from build123d import *

# Parameters (mm, degrees)
SKETCH_1_R          = 2
EXTRUDE_1_DEPTH     = 5
SKETCH_3_W          = 30
SKETCH_3_H          = 2.196813629
EXTRUDE_2_DEPTH     = 10
SKETCH_4_R          = 1.4
CUT_EXTRUDE_2_DEPTH = 20
EXTRUDE_START       = 5.803186371
SKETCH_5_W          = 4
SKETCH_5_H          = 3.6
SKETCH_5_R          = 1.424260765
SKETCH_5_R_2        = 1.4
EXTRUDE_3_DEPTH     = 5.803186371
SKETCH_6_W          = 5.555026764
SKETCH_6_H          = 4.966415056
EXTRUDE_4_DEPTH     = 7
SKETCH_8_R          = 2.9
CUT_EXTRUDE_3_DEPTH = 5
SKETCH_9_R          = 2.2
EXTRUDE_5_DEPTH     = 5
FILLET_1_R          = 1


with BuildPart() as part:
    # 스케치1 → 보스-돌출1 (new, symmetric)
    with BuildSketch(Plane(origin=(0, 0, 0), x_dir=(0, 0, -1), z_dir=(1, 0, 0))):
        Polygon((15, 6.896813629), (-15, 6.896813629), (-15, -1.103186371), (-10.2, -1.103186371), (-10.2, 4.7), (-5, 4.7), (-5, -4), (5, -4), (5, 4.7), (10.2, 4.7), (10.2, -1.103186371), (15, -1.103186371), align=None)
        Circle(SKETCH_1_R, mode=Mode.SUBTRACT)
    extrude(amount=EXTRUDE_1_DEPTH, both=True)

    # 스케치3 → 보스-돌출2 (add, symmetric)
    with BuildSketch(Plane(origin=(0, 0, 0), x_dir=(0, 0, -1), z_dir=(1, 0, 0))):
        with Locations((0, 5.798406814)):
            Rectangle(SKETCH_3_W, SKETCH_3_H)
    extrude(amount=EXTRUDE_2_DEPTH, both=True)

    # 스케치4 → 컷-돌출2 (cut)
    with BuildSketch(Plane(origin=(0, 0, 0), x_dir=(1, 0, 0), z_dir=(0, 1, 0))):
        with Locations(Location((-7, -12, 0), (0, 0, 90))):
            Circle(SKETCH_4_R)
        with Locations(Location((7, -12, 0), (0, 0, 90))):
            Circle(SKETCH_4_R)
        with Locations(Location((7, 12, 0), (0, 0, 90))):
            Circle(SKETCH_4_R)
        with Locations(Location((-7, 12, 0), (0, 0, 90))):
            Circle(SKETCH_4_R)
    extrude(amount=CUT_EXTRUDE_2_DEPTH, mode=Mode.SUBTRACT)

    # 스케치5 → 보스-돌출3 (add)
    # profile 1 of 4: a face of its own
    with BuildSketch(Plane.XZ.offset(-4.7).offset(EXTRUDE_START)):
        with Locations((-7, -12)):
            Rectangle(SKETCH_5_W, SKETCH_5_H)
        with Locations(Location((-7, -12, 0), (0, 0, 90))):
            Circle(SKETCH_5_R, mode=Mode.SUBTRACT)
    # profile 2 of 4: a face of its own
    with BuildSketch(Plane.XZ.offset(-4.7).offset(EXTRUDE_START)):
        with Locations((7, -12)):
            Rectangle(SKETCH_5_W, SKETCH_5_H)
        with Locations(Location((7, -12, 0), (0, 0, 270))):
            Circle(SKETCH_5_R_2, mode=Mode.SUBTRACT)
    # profile 3 of 4: a face of its own
    with BuildSketch(Plane.XZ.offset(-4.7).offset(EXTRUDE_START)):
        with Locations((7, 12)):
            Rectangle(SKETCH_5_W, SKETCH_5_H)
        with Locations(Location((7, 12, 0), (0, 0, 270))):
            Circle(SKETCH_5_R_2, mode=Mode.SUBTRACT)
    # profile 4 of 4: a face of its own
    with BuildSketch(Plane.XZ.offset(-4.7).offset(EXTRUDE_START)):
        with Locations((-7, 12)):
            Rectangle(SKETCH_5_W, SKETCH_5_H)
        with Locations(Location((-7, 12, 0), (0, 0, 270))):
            Circle(SKETCH_5_R_2, mode=Mode.SUBTRACT)
    extrude(amount=-EXTRUDE_3_DEPTH)

    # 스케치6 → 보스-돌출4 (add)
    with BuildSketch(Plane.ZY.offset(5)):
        Rectangle(SKETCH_6_W, SKETCH_6_H)
    extrude(amount=-EXTRUDE_4_DEPTH)

    # 스케치8 → 컷-돌출3 (cut)
    with BuildSketch(Plane.ZY.offset(5)):
        Circle(SKETCH_8_R)
    extrude(amount=-CUT_EXTRUDE_3_DEPTH, mode=Mode.SUBTRACT)

    # 스케치9 → 보스-돌출5 (add)
    with BuildSketch(Plane.ZY):
        Circle(SKETCH_9_R)
    extrude(amount=EXTRUDE_5_DEPTH)

    # 필렛1
    fillet_1_edges = [part.edges().sort_by_distance(p)[0] for p in [
        (-5, 0, -2.2),
    ]]
    fillet(fillet_1_edges, radius=FILLET_1_R)


solid = part.part
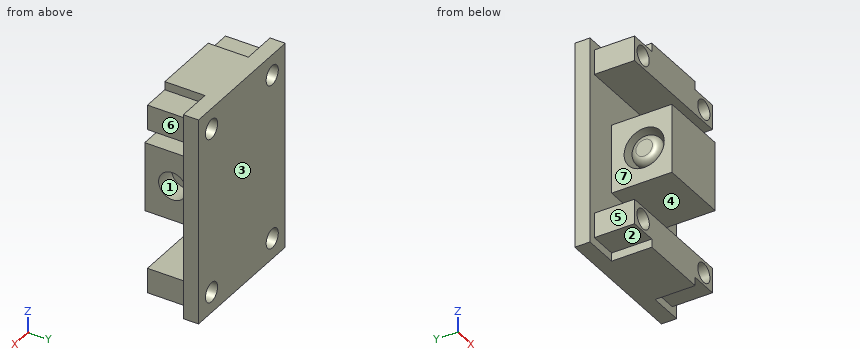
Could you check a few things on this model? Use its own coordinates, in mm. Face numbers are marked on the shaded views. A direction names the side the tool comes from. Round coordinates to 2 decimals unless told otherwise and drop trailing zeros. Order: outer loops, then holes, each group sorted by start corner. A loop starts at its lowest first (then second) coordinate and runs counter-clockwise, first axis right, second up.
(1) Imagine slicing it at A-A (y = 4.25). Write out the boundary of the cut face in (x, z), plus the area to 3 significant figures.
Response values:
outline: (-9, -13.8) - (-5, -13.8) - (-5, -15) - (5, -15) - (5, -13.8) - (9, -13.8) - (9, -10.2) - (-9, -10.2) - close; (-9, 10.2) - (9, 10.2) - (9, 13.8) - (5, 13.8) - (5, 15) - (-5, 15) - (-5, 13.8) - (-9, 13.8) - close; (-5, -5) - (5, -5) - (5, 5) - (-5, 5) - close; hole circle Ø2.85 at (-7, -12); hole circle Ø2.8 at (-7, 12); hole circle Ø2.8 at (7, -12); hole circle Ø2.8 at (7, 12)
area: 229 mm2
(2) I'm going to push flat-ended pins straight in: pin 1 (3.5 mm diameter, centred on y = 0, z = 0, fed in from +X); pin 2 (4.5 mm diameter, centred on y = -0.5, z = 2, fed in from -X); pin 3 (1.1 mm diameter, centred on y = 2, z = -12, fed in from +X); pin 4 (1.5 mm diameter, centred on y = 3, z = 7, fed in from -X). Where does each tip first touch, or does it pass through?
Response values:
pin 1: stops at x = 2
pin 2: stops at x = -5
pin 3: stops at x = 9
pin 4: passes through
(3) If we mould it in two halves opening along Z, with no side actions, what happens to the marked faces 1, 2 and 3? For each: released by +Z, released by -Z, zero draft, split by the parting line, or undercut.
Response values:
face 1: undercut
face 2: released by -Z
face 3: zero draft
(4) Which directions (+Z, -Z, +X, -X, +Y, -Y) give clear straight access to the entire face, cutting with the end or side of a thin tool? Please do the marked faces 4, 5, 6 and 7.
Response values:
face 4: +X, -X, -Y
face 5: +Z, -Z, -X, -Y
face 6: +Z, -Z, +X, -Y
face 7: -X, -Y
(5) Imagine slicing it at D-D (x = -1). Write out the boundary of the cut face in (y, z).
Response values:
outline: (-4, -5) - (4.7, -5) - (4.7, -10.2) - (-1.1, -10.2) - (-1.1, -15) - (6.9, -15) - (6.9, 15) - (-1.1, 15) - (-1.1, 10.2) - (4.7, 10.2) - (4.7, 5) - (-4, 5) - close; circle Ø4.4 at (0, 0); hole circle Ø5.8 at (0, 0)
(6) Please list where these lines run through material, in increasing order: line 1 along X through (y, z) = (0.85, 12); line 2 along Z through (x, y) = (1.25, -1); line 3 along Z through (x, y) = (4.3, 0).
Response values:
line 1: x = -9 to -8.4, -5.6 to 5.6, 8.4 to 9
line 2: z = -15 to -10.2, -5 to 5, 10.2 to 15
line 3: z = -15 to -10.2, -5 to -2, 2 to 5, 10.2 to 15
(7) Imagine slicing it at B-B (x = -7). Count the separate pieces of the cut face and the enclosed holes in it, plus the area to 3 significant figures.
Response values:
separate pieces: 3
enclosed holes: 0
area: 62.6 mm2
